For this review, take the finished solid that the model builds, in its own axes (mm). Round coordinates to 2 decimals unless told otherwise and drop trailing zeros. Order: outer loops, then holes, each group sorted by start corner. A loop starts at its lowest first (then second) coordinate and runs counter-clockwise, first axis right, second up. Notation, with made-up numbers: (2.5, 68.25) - (10.5, 68.25) arc R37 ccw to (10.5, 106.25) - close; hole circle Ø9 at (-11, 61). An arc over 180 degrees is marked (long way). One line per question, with ' | ' between items.
```python
from build123d import *

# Parameters (mm, degrees)
F0_R       = 9.50595
F1_DEPTH   = 990.6
F2_SIZE2   = 0.9165435523
F2_SIZE    = 1.5875
F2_2_SIZE2 = 0.9165435523
F2_2_SIZE  = 1.5875


with BuildPart() as f1:
    # F0 (on Top) → F1 (new body)
    with BuildSketch(Plane.XY):
        Circle(F0_R)
    extrude(amount=-F1_DEPTH)

    # F2
    f2_edges = [f1.edges().sort_by_distance(p)[0] for p in [
        (-9.50595, 0, 0),
    ]]
    f2_side = f1.faces().sort_by_distance((0, 0, 0))[0]
    chamfer(f2_edges, length=F2_SIZE, length2=F2_SIZE2, reference=f2_side)

    # F2#2
    f2_2_edges = [f1.edges().sort_by_distance(p)[0] for p in [
        (-9.50595, 0, -990.6),
    ]]
    f2_2_side = f1.faces().sort_by_distance((0, 0, -990.6))[0]
    chamfer(f2_2_edges, length=F2_2_SIZE, length2=F2_2_SIZE2, reference=f2_2_side)


solid = f1.part
```
(1) We need section A-A on z = -245.5. State the section outline as (x, y) points.
Output values:
outline: circle Ø19.01 at (0, 0)
(2) Insertion check: pin 1 (1.5 mm diameter, centred on x = 7.5, z = -377.5, fed in from +Y); pin 2 (1.5 mm diameter, centred on y = -1.5, z = -205, fed in from +X); pin 3 (2 mm diameter, centred on y = 2, z = -135, fed in from -X). Each pin has a flat end and moves straight along its axis. Give the tip position at first contact, or say it passes through.
Output values:
pin 1: y = 6.69 | pin 2: x = 9.48 | pin 3: x = -9.45
(3) For probe 1 along X at (y, z) = (-1, -668.5); probe 2 along Y at (x, z) = (0.75, -633); probe 3 along X at (y, z) = (-1.25, -446.5), list the stretches that pass through material, from the lowest coordinate up. Write a range as [from, to].
Output values:
probe 1: [-9.45, 9.45] | probe 2: [-9.48, 9.48] | probe 3: [-9.42, 9.42]
